Can you work these out from the drawing? Everything is in mm from the part's minimum corner. Round coordinates to 2 decimals unless told otherwise and drop trailing zeros. Write each loop counter-clockwise with the first axis right and the second up, starting at its lowest first coordinate (ties: lowest second). Pieces come first, ordered by that corner, then holes. Notation, with made-up numbers: (-6, 87) -> (50, 87) arc R15 ccw to (50, 114) -> close; hole circle Ø5 at (-28, 83). An arc over 180 degrees is marked (long way). Put each result on its own line as item: value. Start each with the question number.
1. Suppose I cut it at C-C (y = 0.8). Please give me the cut outline in (x, z).
2. I need wall thicknesses on probe 1 along X at (y, z) = (1.3, 3.85); probe 2 along X at (y, z) = (2.2, 4.5) (1 decimal). Which ranges of each line are inside material? Lowest first, please. Write a range as from..to.
3. We'd pull the mould along Z, two halves only. Please class the marked faces 1, 2 and 3: +Z half, -Z half, draft (parallel to the pull), parting line (faces both ways), or undercut.
4. Suppose I cut it at B-B (x = 3.85). Please give me the cut outline in (y, z).
5. For pin 1 (1.5 mm diameter, centred on y = 1.5, z = 2.5, fed in from -X); pin 2 (1 mm diameter, centred on x = 1.5, y = 2.5, fed in from +Z), each with a flat end and sliding along its axis, tell me the tip position at first contact or that it passes through.
6. Suppose I cut it at A-A (z = 3.85). Please give me the cut outline in (x, y).
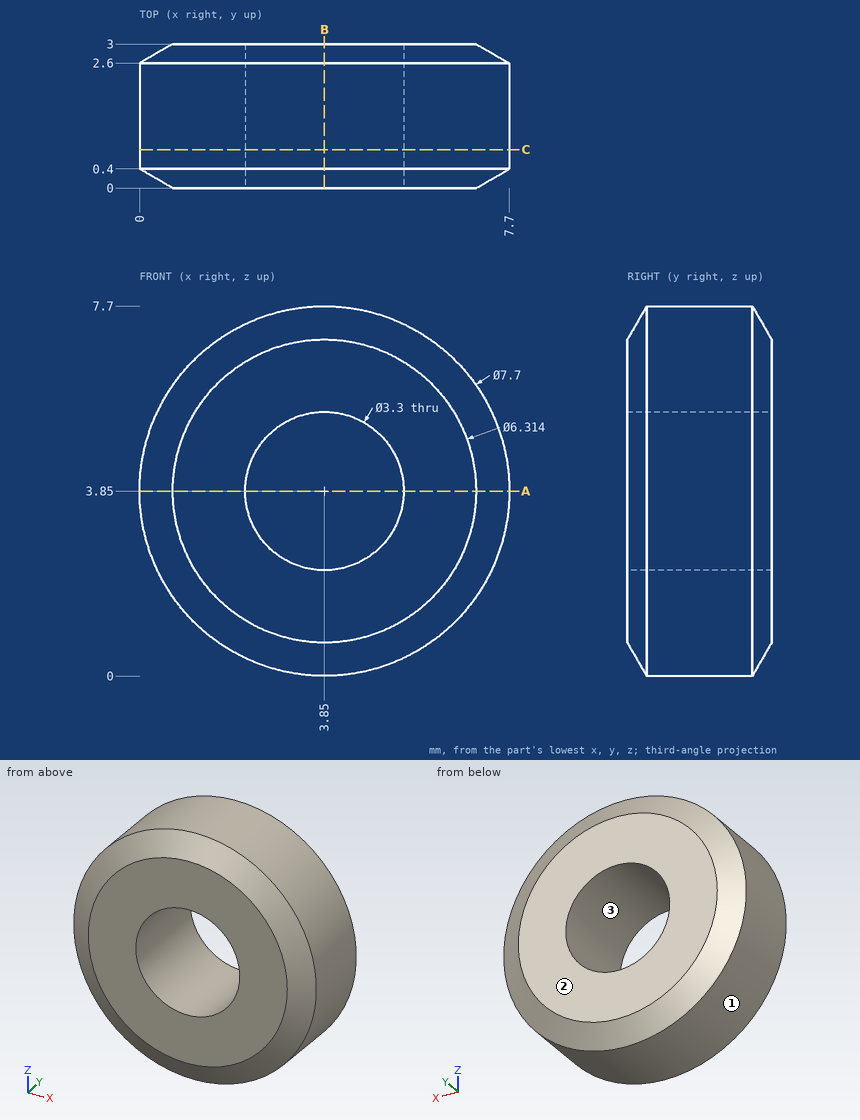
Verdict:
1. outline: circle Ø7.7 at (3.85, 3.85); hole circle Ø3.3 at (3.85, 3.85)
2. probe 1: x = 0..2.2, 5.5..7.7
2. probe 2: x = 0.1..2.3, 5.4..7.6
3. face 1: parting line
3. face 2: draft
3. face 3: undercut
4. outline: (0, 0.69) -> (0.4, 0) -> (2.6, 0) -> (3, 0.69) -> (3, 2.2) -> (0, 2.2) -> close; (0, 5.5) -> (3, 5.5) -> (3, 7.01) -> (2.6, 7.7) -> (0.4, 7.7) -> (0, 7.01) -> close
5. pin 1: stops at x = 0.05
5. pin 2: stops at z = 7.23
6. outline: (0, 0.4) -> (0.69, 0) -> (2.2, 0) -> (2.2, 3) -> (0.69, 3) -> (0, 2.6) -> close; (5.5, 0) -> (7.01, 0) -> (7.7, 0.4) -> (7.7, 2.6) -> (7.01, 3) -> (5.5, 3) -> close
